Solid Edge part; units mm, degrees
sketch "Sketch1" plane through (0, 0, 0) normal (0, -1, 0) x (1, 0, 0)
  line L0 (-30, 30) -> (30, 30)
  line L1 (30, 30) -> (30, -30)
  line L2 (30, -30) -> (-30, -30)
  line L3 (-30, -30) -> (-30, 30)
  dimension "D1" = 30
  dimension "D2" = 30
extrude "Protrusion1" add sketch "Sketch1" along normal mid plane 8
hole "Bohrung_1" at (-20, -4, -20) direction (0, 1, 0) diameter 6.647 end up to next thread major 8 thread length 2
hole "Hole1" at (20, -4, -20) direction (0, 1, 0) diameter 6.647 end up to next thread major 8 thread length 2
hole "Hole2" at (0, -4, 20) direction (0, 1, 0) diameter 6.647 end up to next thread major 8 thread length 2
hole "Bohrung_4" at (7.5, -4, 0) direction (0, 1, 0) diameter 5 end up to next countersink diameter 7 countersink angle 90
hole "Hole3" at (-7.5, -4, 0) direction (0, 1, 0) diameter 5 end up to next countersink diameter 7 countersink angle 90
chamfer "Fase_1" distance 1 angle 45 12 edges at (0, -4, 30) (-30, -4, 0) (30, -4, 0) (30, 4, 0) (30, 0, 30) (0, 4, 30) (-30, 0, 30) (-30, 4, 0) (-30, 0, -30) (0, 4, -30) (0, -4, -30) (30, 0, -30)
chamfer "Fase_2" distance 0.5 angle 45 6 edges at (-3.3235, -4, 20) (0, 4, 16.6765) (16.6765, -4, -20) (20, 4, -23.3235) (-23.3235, -4, -20) (-20, 4, -23.3235)
Check sheet for the modelled part. Datum: model origin and axes. Units: mm. Round coordinates to 2 decimals unless told otherwise and drop trailing zeros. Loops run counter-clockwise (first coordinate to the right, second up) from the corner with the lowest first, then second, coordinate; pieces in that order, holes last. Notation, with made-up numbers: (63.25, 47.5) - (108.25, 47.5) arc R9 cw to (108.25, 54.5) - close; hole circle Ø8 at (-14.5, 51.5). An arc over 180 degrees is marked (long way). Answer as CSV lines item,"result". Start each with the question number.
Item 1: Section check C-C (y = 2). Record the boundary of the cut face in (x, z), and give its area (3 significant figures).
Item 2: Release check for a two-part mould opening along X. For faces 1 (the flat face through (0, 0, -30)), 2 (the cylindrical face through (1, -0.05, 16.83)), 3 (the flat face through (30, 0, 0)) record: +X half, -X half, draft (parallel to the pull), parting line (faces both ways), or undercut.
Item 3: Section check A-A (z = 0). Record the boundary of the cut face in (x, y).
Item 4: Scan lines: line 1 (X direction, y = -0.5, z = 0); line 2 (X direction, y = 0.5, z = -20); line 3 (Z direction, x = 20, y = -1.25). Record each from-to range of solid material in increasing order. Write a range as [from, to].
Item 5: Section check D-D (z = 20). Record the boundary of the cut face in (x, y).
Item 6: Depth check by flat-ended pin: P1, Ø7.5, axis at x = 20, z = -20, coming from the +Y side; P2, Ø6.5, axis at x = 7.5, z = 0, coming from the -Y side; P3, Ø8.5, axis at x = -20, z = -20, coming from the +Y side; P4, Ø7.5, axis at x = 0, z = 20, coming from the -Y side. Enter the tip coordinate at first touch or a pass-through.
Item 7: Section check B-B (x = 20). Record the boundary of the cut face in (y, z), and give its area (3 significant figures).
Report:
1,outline,"(-30, -29) - (-29, -30) - (29, -30) - (30, -29) - (30, 29) - (29, 30) - (-29, 30) - (-30, 29) - close; hole circle Ø6.65 at (-20, -20); hole circle Ø5 at (-7.5, 0); hole circle Ø6.65 at (0, 20); hole circle Ø5 at (7.5, 0); hole circle Ø6.65 at (20, -20)"
1,area,"3,450 mm2"
2,face 1,"draft"
2,face 2,"undercut"
2,face 3,"+X half"
3,outline,"(-30, -3) - (-29, -4) - (-11, -4) - (-10, -3) - (-10, 4) - (-29, 4) - (-30, 3) - close; (-5, -3) - (-4, -4) - (4, -4) - (5, -3) - (5, 4) - (-5, 4) - close; (10, -3) - (11, -4) - (29, -4) - (30, -3) - (30, 3) - (29, 4) - (10, 4) - close"
4,line 1,"x = [-30, -10], [-5, 5], [10, 30]"
4,line 2,"x = [-30, -23.32], [-16.68, 16.68], [23.32, 30]"
4,line 3,"z = [-30, -23.32], [-16.68, 30]"
5,outline,"(-30, -3) - (-29, -4) - (-3.82, -4) - (-3.32, -3.5) - (-3.32, 3.5) - (-3.82, 4) - (-29, 4) - (-30, 3) - close; (3.32, -3.5) - (3.82, -4) - (29, -4) - (30, -3) - (30, 3) - (29, 4) - (3.82, 4) - (3.32, 3.5) - close"
6,P1,"stops at y = 3.93"
6,P2,"stops at y = -3.75"
6,P3,"stops at y = 4"
6,P4,"stops at y = -3.93"
7,outline,"(-4, -29) - (-3, -30) - (3, -30) - (4, -29) - (4, -23.82) - (3.5, -23.32) - (-3.5, -23.32) - (-4, -23.82) - close; (-4, -16.18) - (-3.5, -16.68) - (3.5, -16.68) - (4, -16.18) - (4, 29) - (3, 30) - (-3, 30) - (-4, 29) - close"
7,area,"424 mm2"
